The model under review builds one solid part; all positions refer to its coordinate system, in mm. A direction names the side the tool comes from. Give positions to 0.01 mm unless a question says otherwise; leave off trailing zeros. Order: outer loops, then holes, each group sorted by start corner. A loop starts at its lowest first (then second) coordinate and runs counter-clockwise, first axis right, second up. Notation, with made-up numbers: (-33.75, -35) -> (-13.75, -35) arc R6 cw to (-13.75, -27) -> close; hole circle Ø4 at (42.5, -38.75). An arc over 180 degrees is marked (long way). Use one line per item in the form item = value.
```python
from build123d import *

# Parameters (mm, degrees)
SKETCH3_W              = 111
SKETCH3_H              = 75
SKETCH3_R              = 8.25
WELL_LIGHT_GUIDE_DEPTH = 10
SKETCH1_R              = 2.5
PCB_MOUNT_PLATE_DEPTH  = 2.5
SKETCH4_W              = 10
SKETCH4_H              = 2
SKETCH4_W_2            = 2
SKETCH4_H_2            = 10
TOP_GUIDE_TABS_DEPTH   = 12
SKETCH5_W              = 10
SKETCH5_H              = 0.4
SKETCH5_W_2            = 0.4
SKETCH5_H_2            = 10
F_3DPRINT_SPACER_DEPTH = 158.95766838
FILLET1_R              = 10


with BuildPart() as part:
    # Sketch3 → Well light guide (new body)
    with BuildSketch(Plane(origin=(0, 0, 0), x_dir=(1, 0, 0), z_dir=(0, 1, 0))):
        with Locations((64, 43)):
            Rectangle(SKETCH3_W, SKETCH3_H)
        with Locations(Location((19, 70, 0), (0, 0, 270))):
            Circle(SKETCH3_R, mode=Mode.SUBTRACT)
        with Locations(Location((37, 70, 0), (0, 0, 270))):
            Circle(SKETCH3_R, mode=Mode.SUBTRACT)
        with Locations(Location((55, 70, 0), (0, 0, 270))):
            Circle(SKETCH3_R, mode=Mode.SUBTRACT)
        with Locations(Location((73, 70, 0), (0, 0, 270))):
            Circle(SKETCH3_R, mode=Mode.SUBTRACT)
        with Locations(Location((91, 70, 0), (0, 0, 270))):
            Circle(SKETCH3_R, mode=Mode.SUBTRACT)
        with Locations(Location((109, 70, 0), (0, 0, 270))):
            Circle(SKETCH3_R, mode=Mode.SUBTRACT)
        with Locations(Location((37, 52, 0), (0, 0, 270))):
            Circle(SKETCH3_R, mode=Mode.SUBTRACT)
        with Locations(Location((55, 52, 0), (0, 0, 270))):
            Circle(SKETCH3_R, mode=Mode.SUBTRACT)
        with Locations(Location((73, 52, 0), (0, 0, 270))):
            Circle(SKETCH3_R, mode=Mode.SUBTRACT)
        with Locations(Location((91, 52, 0), (0, 0, 270))):
            Circle(SKETCH3_R, mode=Mode.SUBTRACT)
        with Locations(Location((109, 52, 0), (0, 0, 270))):
            Circle(SKETCH3_R, mode=Mode.SUBTRACT)
        with Locations(Location((37, 34, 0), (0, 0, 270))):
            Circle(SKETCH3_R, mode=Mode.SUBTRACT)
        with Locations(Location((55, 34, 0), (0, 0, 270))):
            Circle(SKETCH3_R, mode=Mode.SUBTRACT)
        with Locations(Location((73, 34, 0), (0, 0, 270))):
            Circle(SKETCH3_R, mode=Mode.SUBTRACT)
        with Locations(Location((91, 34, 0), (0, 0, 270))):
            Circle(SKETCH3_R, mode=Mode.SUBTRACT)
        with Locations(Location((109, 34, 0), (0, 0, 270))):
            Circle(SKETCH3_R, mode=Mode.SUBTRACT)
        with Locations(Location((37, 16, 0), (0, 0, 270))):
            Circle(SKETCH3_R, mode=Mode.SUBTRACT)
        with Locations(Location((55, 16, 0), (0, 0, 270))):
            Circle(SKETCH3_R, mode=Mode.SUBTRACT)
        with Locations(Location((73, 16, 0), (0, 0, 270))):
            Circle(SKETCH3_R, mode=Mode.SUBTRACT)
        with Locations(Location((91, 16, 0), (0, 0, 270))):
            Circle(SKETCH3_R, mode=Mode.SUBTRACT)
        with Locations(Location((109, 16, 0), (0, 0, 270))):
            Circle(SKETCH3_R, mode=Mode.SUBTRACT)
        with Locations(Location((19, 52, 0), (0, 0, 270))):
            Circle(SKETCH3_R, mode=Mode.SUBTRACT)
        with Locations(Location((19, 34, 0), (0, 0, 270))):
            Circle(SKETCH3_R, mode=Mode.SUBTRACT)
        with Locations(Location((19, 16, 0), (0, 0, 270))):
            Circle(SKETCH3_R, mode=Mode.SUBTRACT)
    extrude(amount=WELL_LIGHT_GUIDE_DEPTH)

    # Sketch1 → PCB mount plate (add)
    # profile 1 of 4: a face of its own
    with BuildSketch(Plane(origin=(0, 0, 0), x_dir=(1, 0, 0), z_dir=(0, 1, 0))):
        with BuildLine():
            Line((116.75, 84), (116.75, 80.5))
            Line((116.75, 80.5), (119.5, 80.5))
            Line((119.5, 80.5), (119.5, 77.75))
            Line((119.5, 77.75), (123, 77.75))
            ThreePointArc((123, 77.75), (127.419417382, 88.419417382), (116.75, 84))
        make_face()
        with Locations(Location((123, 84, 0), (0, 0, 270))):
            Circle(SKETCH1_R, mode=Mode.SUBTRACT)
    # profile 2 of 4: a face of its own
    with BuildSketch(Plane(origin=(0, 0, 0), x_dir=(1, 0, 0), z_dir=(0, 1, 0))):
        with BuildLine():
            Line((11.25, 84), (11.25, 80.5))
            Line((11.25, 80.5), (8.5, 80.5))
            Line((8.5, 80.5), (8.5, 77.75))
            Line((8.5, 77.75), (5, 77.75))
            ThreePointArc((5, 77.75), (0.580582618, 88.419417382), (11.25, 84))
        make_face()
        with Locations(Location((5, 84, 0), (0, 0, 90))):
            Circle(SKETCH1_R, mode=Mode.SUBTRACT)
    # profile 3 of 4: a face of its own
    with BuildSketch(Plane(origin=(0, 0, 0), x_dir=(1, 0, 0), z_dir=(0, 1, 0))):
        with BuildLine():
            Line((11.25, 2), (11.25, 5.5))
            Line((11.25, 5.5), (8.5, 5.5))
            Line((8.5, 5.5), (8.5, 8.25))
            Line((8.5, 8.25), (5, 8.25))
            ThreePointArc((5, 8.25), (0.580582618, -2.419417382), (11.25, 2))
        make_face()
        with Locations(Location((5, 2, 0), (0, 0, 270))):
            Circle(SKETCH1_R, mode=Mode.SUBTRACT)
    # profile 4 of 4: a face of its own
    with BuildSketch(Plane(origin=(0, 0, 0), x_dir=(1, 0, 0), z_dir=(0, 1, 0))):
        with BuildLine():
            Line((119.5, 5.5), (116.75, 5.5))
            Line((116.75, 5.5), (116.75, 2))
            ThreePointArc((116.75, 2), (127.419417382, -2.419417382), (123, 8.25))
            Line((123, 8.25), (119.5, 8.25))
            Line((119.5, 8.25), (119.5, 5.5))
        make_face()
        with Locations(Location((123, 2, 0), (0, 0, 90))):
            Circle(SKETCH1_R, mode=Mode.SUBTRACT)
    extrude(amount=PCB_MOUNT_PLATE_DEPTH)

    # Sketch4 → Top guide tabs (add)
    with BuildSketch(Plane.XZ):
        with Locations((39, -81.5)):
            Rectangle(SKETCH4_W, SKETCH4_H)
        with Locations((89, -4.5)):
            Rectangle(SKETCH4_W, SKETCH4_H)
        with Locations((7.5, -28)):
            Rectangle(SKETCH4_W_2, SKETCH4_H_2)
        with Locations((120.5, -58)):
            Rectangle(SKETCH4_W_2, SKETCH4_H_2)
        with Locations((39, -4.5)):
            Rectangle(SKETCH4_W, SKETCH4_H)
        with Locations((89, -81.5)):
            Rectangle(SKETCH4_W, SKETCH4_H)
    extrude(amount=-TOP_GUIDE_TABS_DEPTH)

    # Sketch5 → 3Dprint spacer (cut, through all)
    with BuildSketch(Plane(origin=(0, 10, 0), x_dir=(1, 0, 0), z_dir=(0, 1, 0))):
        with Locations((89, 80.7)):
            Rectangle(SKETCH5_W, SKETCH5_H)
        with Locations((89, 5.3)):
            Rectangle(SKETCH5_W, SKETCH5_H)
        with Locations((119.7, 58)):
            Rectangle(SKETCH5_W_2, SKETCH5_H_2)
        with Locations((39, 80.7)):
            Rectangle(SKETCH5_W, SKETCH5_H)
        with Locations((39, 5.3)):
            Rectangle(SKETCH5_W, SKETCH5_H)
        with Locations((8.3, 28)):
            Rectangle(SKETCH5_W_2, SKETCH5_H_2)
    extrude(amount=F_3DPRINT_SPACER_DEPTH, mode=Mode.SUBTRACT)

    # Fillet1
    # the kernel refuses this fillet: 10 mm, written as the material it adds along each edge
    with BuildSketch(Plane(origin=(116.75, 0, -80.5), x_dir=(0.0866364142554912, 0, -0.9962399970513885), z_dir=(0, 1, 0)), Plane(origin=(119.5, 0, -8.25), x_dir=(0.9962399970513889, 0, 0.08663641425548835), z_dir=(0, 1, 0)), Plane(origin=(8.5, 0, -77.75), x_dir=(-0.9962399970513889, 0, -0.08663641425548864), z_dir=(0, 1, 0))) as fillet1_piece_1:
        with BuildLine():
            CenterArc((9.213569299, 9.477236051), FILLET1_R, 184.970131688, 66.421821522)
            Line((-0.748830671, 8.610871908), (-1.745070668, 8.524235494))
            Line((-1.745070668, 8.524235494), (-0.996239997, -0.086636414))
            Line((-0.996239997, -0.086636414), (0.086636414, -0.996239997))
            ThreePointArc((0.086636414, -0.996239997), (3.573476404, -0.693012547), (5.70355275, -0.947723605))
            Line((5.70355275, -0.947723605), (6.022645164, 0))
        make_face()
    extrude(amount=2.5)
    with BuildSketch(Plane(origin=(119.5, 0, -77.75), x_dir=(0, 0, 1), z_dir=(0, 1, 0)), Plane(origin=(116.75, 0, -5.5), x_dir=(-1, 0, 0), z_dir=(0, 1, 0)), Plane(origin=(8.5, 0, -8.25), x_dir=(0, 0, -1), z_dir=(0, 1, 0)), Plane(origin=(11.25, 0, -80.5), x_dir=(1, 0, 0), z_dir=(0, 1, 0))) as fillet1_piece_2:
        with BuildLine():
            CenterArc((8.643371009, 10), FILLET1_R, 203.578178478, 66.421821522)
            Line((-0.521780381, 6), (-1.43829552, 5.6))
            ThreePointArc((-1.43829552, 5.6), (-1, 3.5), (-1, 0))
            Line((-1, 0), (0, -1))
            Line((0, -1), (8.643371009, -1))
            Line((8.643371009, -1), (8.643371009, 0))
        make_face()
    extrude(amount=2.5)
    with BuildSketch(Plane(origin=(11.25, 0, -5.5), x_dir=(1, 0, 0), z_dir=(0, 1, 0))) as fillet1_piece_3:
        with BuildLine():
            CenterArc((8.643371009, -10), FILLET1_R, 90, 66.421821522)
            Line((-0.521780381, -6), (-1.43829552, -5.6))
            ThreePointArc((-1.43829552, -5.6), (-1, -3.5), (-1, 0))
            Line((-1, 0), (0, 1))
            Line((0, 1), (8.643371009, 1))
            Line((8.643371009, 1), (8.643371009, 0))
        make_face()
    extrude(amount=2.5)


solid = part.part
```
1. Add section D-D on x = 123. Give the boundary of the cut face in (y, z).
Values:
outline = (0, -90.25) -> (2.5, -90.25) -> (2.5, -86.5) -> (0, -86.5) -> close; (0, -81.5) -> (2.5, -81.5) -> (2.5, -76.71) -> (0, -76.71) -> close; (0, -9.29) -> (2.5, -9.29) -> (2.5, -4.5) -> (0, -4.5) -> close; (0, 0.5) -> (2.5, 0.5) -> (2.5, 4.25) -> (0, 4.25) -> close
2. The part is to be moulded in two halves that separate along X. For faces 1 (the face through (100.946, 4.93, -53.788)), 2 (the face through (119.5, 5, -29)), 3 (the face through (8.5, 6, -14)), 4 (the face through (82.946, 4.93, -53.788)), say which applies: +X half, -X half, draft (parallel to the pull), parting line (faces both ways), or undercut.
Values:
face_1 = undercut
face_2 = +X half
face_3 = -X half
face_4 = undercut
3. For pin 1 Ø3 at (x, y) = (104, 4.5) entering from -Z; pin 2 Ø5 at (y, z) = (6, -8) entering from +X; pin 3 Ø0.6 at (y, z) = (5.5, -81.5) entering from -X; pin 4 Ø6 at (x, z) = (34.5, -17.5) entering from -Y, all flat-tipped, find the tip position at first contact; note any pin that passes through.
Values:
pin_1 = -80.5
pin_2 = 119.5
pin_3 = 34
pin_4 = through
4. Add section B-B on z = -45.5. Give the boundary of the cut face in (x, y).
Values:
outline = (8.5, 0) -> (13.92, 0) -> (13.92, 10) -> (8.5, 10) -> close; (24.08, 0) -> (31.92, 0) -> (31.92, 10) -> (24.08, 10) -> close; (42.08, 0) -> (49.92, 0) -> (49.92, 10) -> (42.08, 10) -> close; (60.08, 0) -> (67.92, 0) -> (67.92, 10) -> (60.08, 10) -> close; (78.08, 0) -> (85.92, 0) -> (85.92, 10) -> (78.08, 10) -> close; (96.08, 0) -> (103.92, 0) -> (103.92, 10) -> (96.08, 10) -> close; (114.08, 0) -> (119.5, 0) -> (119.5, 10) -> (114.08, 10) -> close
5. For L1, parallel to Z at x = 42, y = 11.5; L2, parallel to Z at x = 61.5, y = 1.5; L3, parallel to Z at x = 87, y = 8, list the stretches that pass through material, from the lowest coordinate up.
Values:
L1 = -82.5 to -80.9, -5.1 to -3.5
L2 = -80.5 to -75.08, -64.92 to -57.08, -46.92 to -39.08, -28.92 to -21.08, -10.92 to -5.5
L3 = -82.5 to -77.22, -62.78 to -59.22, -44.78 to -41.22, -26.78 to -23.22, -8.78 to -3.5
6. Add section C-C on y = 7.5. Count the separate pieces of the cut face and the enclosed holes in it, then the cut area to 3 significant figures.
Values:
separate_pieces = 1
enclosed_holes = 24
area = 3,310 mm^2
7. Tool access review of faces 5 (the face through (6.91, 1.23, -74.52)), 6 (the face through (107, 5, -5.5)), 7 (the face through (121.178, 1.232, -74.652)), 8 (the face through (64.946, 4.93, -53.788)): name each direction out of +Z, -Z, +X, -X, +Y, -Y from which nothing blocks a thin tool from reaching the whole face with its end or side.
Values:
face_5 = -X, +Y, -Y
face_6 = +Z, +Y
face_7 = +X, +Y, -Y
face_8 = +Y, -Y
8. Add section A-A on x = 37. Give the boundary of the cut face in (y, z).
Values:
outline = (0, -82.5) -> (12, -82.5) -> (12, -80.9) -> (10, -80.9) -> (10, -78.25) -> (0, -78.25) -> close; (0, -61.75) -> (10, -61.75) -> (10, -60.25) -> (0, -60.25) -> close; (0, -43.75) -> (10, -43.75) -> (10, -42.25) -> (0, -42.25) -> close; (0, -25.75) -> (10, -25.75) -> (10, -24.25) -> (0, -24.25) -> close; (0, -7.75) -> (10, -7.75) -> (10, -5.1) -> (12, -5.1) -> (12, -3.5) -> (0, -3.5) -> close
